Here's how the part is built. I have some questions about the finished solid (model axes, mm). Face numbers are marked on the shaded views. Coordinates: 2 decimals unless noted, no trailing zeros. Write each loop counter-clockwise with the first axis right and the second up, starting at its lowest first coordinate (ties: lowest second). Pieces come first, ordered by that corner, then holes. Notation, with made-up numbers: (-14.75, 33) -> (11.25, 33) arc R23 cw to (11.25, 65) -> close; hole circle Ø8 at (-29.5, -9.5). An arc over 180 degrees is marked (long way). Use a Markdown table: item, result. Add a question column.
Autodesk Inventor part; units mm, degrees
ref_plane "YZ Plane" through (0, 0, 0) normal (1, 0, 0) x (0, 1, 0)
ref_plane "XZ Plane" through (0, 0, 0) normal (0, 1, 0) x (-1, 0, 0)
ref_plane "XY Plane" through (0, 0, 0) normal (0, 0, 1) x (1, 0, 0)
sketch "Sketch1" plane through (0, 0, 0) normal (0, 0, 1) x (1, 0, 0)
  line L0 (-27.5, -6.5) -> (27.5, -6.5)
  line L1 (27.5, -6.5) -> (27.5, 6.5)
  line L2 (27.5, 6.5) -> (-27.5, 6.5)
  line L3 (-27.5, 6.5) -> (-27.5, -6.5)
  line L4 (-27.5, -6.5) -> (27.5, 6.5) construction
  line L5 (27.5, -6.5) -> (-27.5, 6.5) construction
  circle A0 centre (-21, 0) radius 2.5
  circle A1 centre (21, 0) radius 2.5
  point P0 (0, 0)
  dimension "d0" = 55
  dimension "d1" = 13
  dimension "d2" = 5
  dimension "d3" = 5
  dimension "d4" = 42
  dimension "d5" = 21
  dimension "d6" = 6.5
  dimension "d7" = 6.5
extrude "Extrusion1" add sketch "Sketch1" along normal blind 7
fillet "Fillet1" radius 2 4 edges at (27.5, 6.5, 3.5) (27.5, -6.5, 3.5) (-27.5, 6.5, 3.5) (-27.5, -6.5, 3.5)
properties part number "dem bac dan"
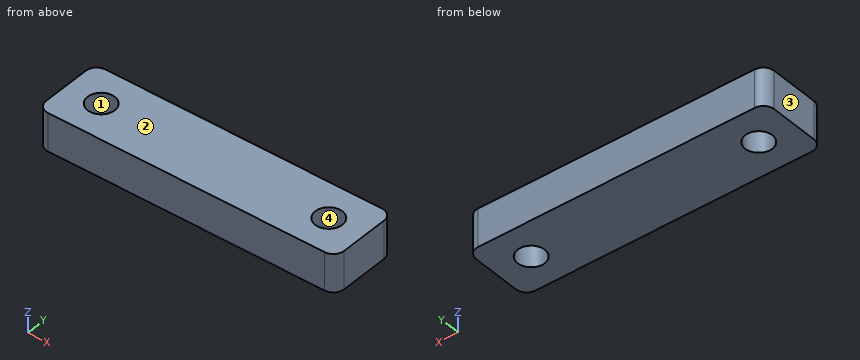
Q1. Please list where these lines run through material, in increasing order: line 1 (Y direction, x = -21, z = 2); line 2 (X direction, y = 0.5, z = 5.25); line 3 (X direction, y = 1, z = 3).
Q2. Suppose I cut it at A-A, the plane y = 1.5. Write out the boundary of the cut face in (x, z).
Q3. Suppose I cut it at D-D, the plane y = 5.75. Write out the boundary of the cut face in (x, z), and give its area (3 significant figures).
Q4. Suppose I cut it at C-C, the plane z = 5. Write out the boundary of the cut face in (x, y), and give its area (3 significant figures).
Q5. Suppose I cut it at B-B, the plane x = 21. Write out the boundary of the cut face in (y, z).
Q6. Thinking about a two-plate mould opening in X: for the marked faces 1, 2, 3 and 4, which applies, released by +X, released by -X, zero draft, split by the parting line, or undercut?
Answer key:
| question | item | result |
|---|---|---|
| 1 | line 1 | y = -6.5 to -2.5, 2.5 to 6.5 |
| 1 | line 2 | x = -27.5 to -23.45, -18.55 to 18.55, 23.45 to 27.5 |
| 1 | line 3 | x = -27.5 to -23.29, -18.71 to 18.71, 23.29 to 27.5 |
| 2 | outline | (-27.5, 0) -> (-23, 0) -> (-23, 7) -> (-27.5, 7) -> close; (-19, 0) -> (19, 0) -> (19, 7) -> (-19, 7) -> close; (23, 0) -> (27.5, 0) -> (27.5, 7) -> (23, 7) -> close |
| 3 | outline | (-27.06, 0) -> (27.06, 0) -> (27.06, 7) -> (-27.06, 7) -> close |
| 3 | area | 379 mm^2 |
| 4 | outline | (-27.5, -4.5) arc R2 ccw to (-25.5, -6.5) -> (25.5, -6.5) arc R2 ccw to (27.5, -4.5) -> (27.5, 4.5) arc R2 ccw to (25.5, 6.5) -> (-25.5, 6.5) arc R2 ccw to (-27.5, 4.5) -> close; hole circle Ø5 at (-21, 0); hole circle Ø5 at (21, 0) |
| 4 | area | 672 mm^2 |
| 5 | outline | (-6.5, 0) -> (-2.5, 0) -> (-2.5, 7) -> (-6.5, 7) -> close; (2.5, 0) -> (6.5, 0) -> (6.5, 7) -> (2.5, 7) -> close |
| 6 | face 1 | undercut |
| 6 | face 2 | zero draft |
| 6 | face 3 | released by -X |
| 6 | face 4 | undercut |
